Read the model definition and answer for the solid it produces. Units are mm, in the model's axes. A direction names the side the tool comes from. Coordinates: 2 decimals unless noted, no trailing zeros. Write each loop counter-clockwise with the first axis right and the second up, starting at its lowest first coordinate (ties: lowest second). Pieces come first, ordered by that corner, then holes. Notation, with made-up numbers: (46, 59) - (85, 59) arc R11 ccw to (85, 74) - close; hole circle Ø2 at (-25.75, 33). An arc over 180 degrees is marked (long way). Return JSON: item names as keys, results as strings.
```python
from build123d import *

# Parameters (mm, degrees)
SKETCH1_R           = 14
SKETCH1_R_2         = 1.6
SKETCH1_R_3         = 4.25
BOSS_EXTRUDE1_DEPTH = 26
CHAMFER1_SIZE       = 2
SKETCH2_R           = 14
BOSS_EXTRUDE2_DEPTH = 1
CHAMFER2_SIZE       = 2
SKETCH4_R           = 1.5
BOSS_EXTRUDE3_DEPTH = 13


with BuildPart() as part:
    # Sketch1 → Boss-Extrude1 (new body)
    with BuildSketch(Plane(origin=(0, 0, 0), x_dir=(1, 0, 0), z_dir=(0, 1, 0))):
        with Locations(Location((0, 0, 0), (0, 0, 90))):
            Circle(SKETCH1_R)
        with Locations(Location((-6.717514421, 6.717514421, 0), (0, 0, 90))):
            Circle(SKETCH1_R_2, mode=Mode.SUBTRACT)
        with Locations(Location((5.656854249, 5.656854249, 0), (0, 0, 90))):
            Circle(SKETCH1_R_2, mode=Mode.SUBTRACT)
        with Locations(Location((0, 0, 0), (0, 0, 90))):
            Circle(SKETCH1_R_3, mode=Mode.SUBTRACT)
        with Locations(Location((6.717514421, -6.717514421, 0), (0, 0, 90))):
            Circle(SKETCH1_R_2, mode=Mode.SUBTRACT)
        with Locations(Location((-5.656854249, -5.656854249, 0), (0, 0, 90))):
            Circle(SKETCH1_R_2, mode=Mode.SUBTRACT)
    extrude(amount=BOSS_EXTRUDE1_DEPTH)

    # Chamfer1
    chamfer1_edges = [part.edges().sort_by_distance(p)[0] for p in [
        (0, 0, 14),
    ]]
    chamfer(chamfer1_edges, length=CHAMFER1_SIZE)

    # Sketch2 → Boss-Extrude2 (add)
    with BuildSketch(Plane(origin=(0, 26, 0), x_dir=(1, 0, 0), z_dir=(0, 1, 0))):
        with Locations(Location((0, 0, 0), (0, 0, 90))):
            Circle(SKETCH2_R)
    extrude(amount=BOSS_EXTRUDE2_DEPTH)

    # Chamfer2
    chamfer2_edges = [part.edges().sort_by_distance(p)[0] for p in [
        (0, 27, 14),
    ]]
    chamfer(chamfer2_edges, length=CHAMFER2_SIZE)

    # Sketch4 → Boss-Extrude3 (add)
    with BuildSketch(Plane(origin=(0, 27, 0), x_dir=(1, 0, 0), z_dir=(0, 1, 0))):
        with Locations(Location((0, 0, 0), (0, 0, 90))):
            Circle(SKETCH4_R)
    extrude(amount=BOSS_EXTRUDE3_DEPTH)


solid = part.part
```
(1) A cutting plane is placed at B-B (z = 0). Determine the outline of the cut face in (x, y).
Answer:
{"outline": "(-14, 2) - (-12, 0) - (-4.25, 0) - (-4.25, 26) - (4.25, 26) - (4.25, 0) - (12, 0) - (14, 2) - (14, 25) - (12, 27) - (1.5, 27) - (1.5, 40) - (-1.5, 40) - (-1.5, 27) - (-12, 27) - (-14, 25) - close"}
(2) A cutting plane is placed at C-C (y = 21). Determine the outline of the cut face in (x, z).
Answer:
{"outline": "circle Ø28 at (0, 0); hole circle Ø3.2 at (-6.72, -6.72); hole circle Ø3.2 at (-5.66, 5.66); hole circle Ø8.5 at (0, 0); hole circle Ø3.2 at (5.66, -5.66); hole circle Ø3.2 at (6.72, 6.72)"}
(3) Which of the six approach directions +Z, -Z, +X, -X, +Y, -Y give full straight-line access (tool end or side, diameter ignored) to faces 4 (the face through (13.67, 13.34, 3.03)), 5 (the face through (7, 26, 7))?
Answer:
{"face 4": "+Y, -Y", "face 5": "-Y"}
(4) Straight lines are drawn through the part: line 1 (X direction, y = 17, z = 0); line 2 (X direction, y = 2.5, z = -6.75); line 3 (Y direction, x = 8, z = 7.75). For each, find the intervals that lie inside material, in ascending order. Write a range as from..to.
Answer:
{"line 1": "-14..-4.25, 4.25..14", "line 2": "-12.27..-8.32, -5.12..4.49, 6.83..12.27", "line 3": "0..27"}
(5) A cutting plane is placed at A-A (x = 0). Determine the outline of the cut face in (y, z), and give its area (3 significant figures).
Answer:
{"outline": "(0, -12) - (2, -14) - (25, -14) - (27, -12) - (27, -1.5) - (40, -1.5) - (40, 1.5) - (27, 1.5) - (27, 12) - (25, 14) - (2, 14) - (0, 12) - (0, 4.25) - (26, 4.25) - (26, -4.25) - (0, -4.25) - close", "area": "566 mm²"}
(6) Flat-ended cylindrical pins translate along their axes: P1, Ø2, axis at x = 5.5, z = -1, coming from the +Y side; P2, Ø4, axis at x = 0.5, z = -2, coming from the -Y side; P3, Ø4, axis at x = -9, y = 11.5, coming from the -Z side. Find the tip coordinate at first contact, or state that the pin passes through.
Answer:
{"P1": "y = 27", "P2": "y = 26", "P3": "z = -12.12"}
(7) Determine the mould class of faces 1 (the face through (0, 26, 0)), 2 (the face through (0, 40, 0)), 3 (the face through (-0.45, 33.41, -1.43)) for opening direction Z: +Z half, -Z half, draft (parallel to the pull), parting line (faces both ways), or undercut.
Answer:
{"face 1": "undercut", "face 2": "draft", "face 3": "parting line"}
